Input: dimensioned drawing with shaded views. Units: mm. Origin: part minimum x, y, z. A direction names the side the tool comes from. Give positions to 0.01 mm unless a question says otherwise; leave off trailing zeros. Order: outer loops, then holes, each group sorted by start corner. A loop starts at its lowest first (then second) coordinate and runs counter-clockwise, first axis right, second up. Notation, with made-up numbers: M 59.25,71.5 L 118.25,71.5 A12 cw 118.25,84.5 Z; hole C 12,56 d8. An arc over 180 degrees is marked long. Answer in a Markdown table with one row per item. Add a question column.
(1) Mould query, pull axis Y, two halves, no side actions, for the marked faces 4, 5 and 6. Classes: pulls with the +Y half, pulls with the -Y half, needs draft (parallel to the pull), parting line crosses it, or undercut.
(2) Material intervals for line 1 along Y through (x, z) = (28, 0.5); line 2 along Z through (x, y) = (38, 12.5); line 3 along X through (y, z) = (6, 5.75), sorted ascending.
(3) Pin query (flat end, axial travel): P1, Ø1.5, axis at y = 3, z = 3, coming from the -X side. Return the tip coordinate at first contact, or that it passes through.
(4) Section query B-B, the plane x = 27.5. Return loops of the section in (y, z), plus the area to 3 significant figures.
(5) Set-up query: the marked faces 1, 2 and 3. Return all of +Z, -Z, +X, -X, +Y, -Y with unobstructed straight access to the full face (end or side cutting, diameter ignored); none if empty.
(6) Section query A-A, the plane y = 11. Return loops of the section in (x, z).
(7) Section query C-C, the plane z = 1.25. Return loops of the section in (x, y).
(8) Section query D-D, the plane y = 18.5. Return loops of the section in (x, z), plus the area to 3 significant figures.
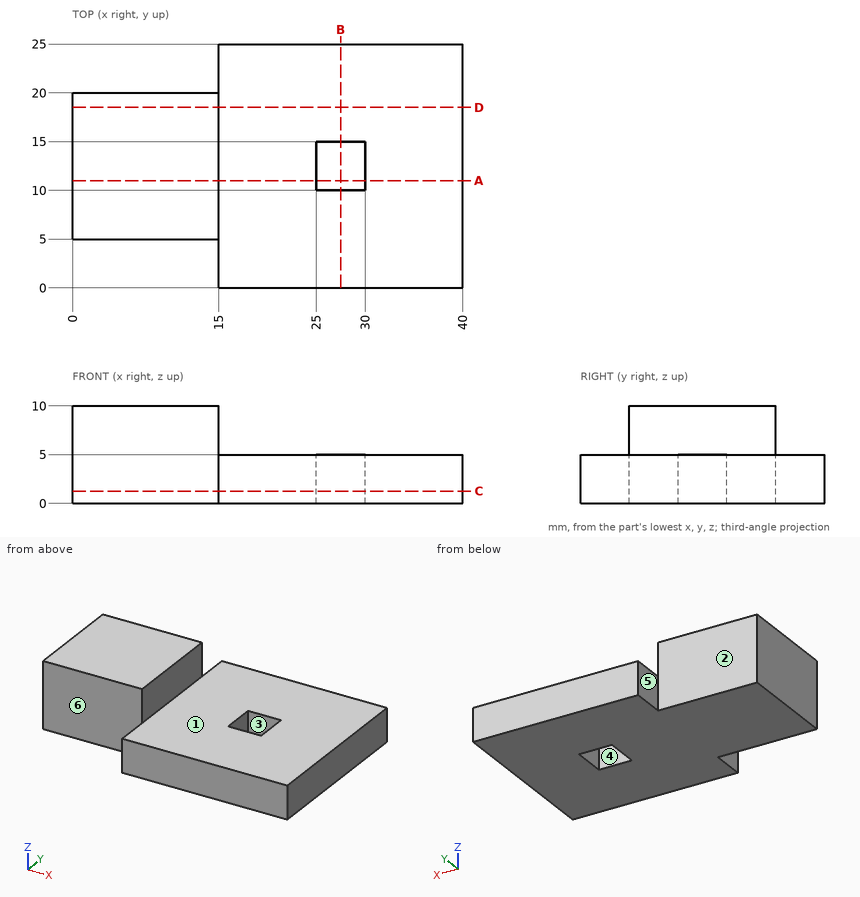
Values follow:
| question | item | result |
|---|---|---|
| 1 | face 4 | undercut |
| 1 | face 5 | needs draft |
| 1 | face 6 | pulls with the -Y half |
| 2 | line 1 | y = 0 to 10, 15 to 25 |
| 2 | line 2 | z = 0 to 5 |
| 2 | line 3 | x = 0 to 15 |
| 3 | P1 | stops at x = 15 |
| 4 | outline | M 0,0 L 10,0 L 10,5 L 0,5 Z; M 15,0 L 25,0 L 25,5 L 15,5 Z |
| 4 | area | 100 mm² |
| 5 | face 1 | +Z, +X, +Y, -Y |
| 5 | face 2 | +Z, -Z, -X, +Y |
| 5 | face 3 | +Z, -Z |
| 6 | outline | M 0,0 L 25,0 L 25,5 L 15,5 L 15,10 L 0,10 Z; M 30,0 L 40,0 L 40,5 L 30,5 Z |
| 7 | outline | M 0,5 L 15,5 L 15,0 L 40,0 L 40,25 L 15,25 L 15,20 L 0,20 Z; hole M 25,10 L 30,10 L 30,15 L 25,15 Z |
| 8 | outline | M 0,0 L 40,0 L 40,5 L 15,5 L 15,10 L 0,10 Z |
| 8 | area | 275 mm² |
